```python
from build123d import *

# Parameters (mm, degrees)
SALIENTE_EXTRUIR1_DEPTH = 400
REDONDEO1_R             = 0.5
CROQUIS2_R              = 2
CROQUIS2_R_2            = 1.75
CORTAR_EXTRUIR1_DEPTH   = 16


with BuildPart() as part:
    # Croquis1 → Saliente-Extruir1 (new body)
    with BuildSketch(Plane.XY):
        Polygon((-7.5, 15), (-7.5, 0), (7.5, 0), (7.5, 15), (5.5, 15), (5.5, 2), (-5.5, 2), (-5.5, 15), align=None)
    extrude(amount=SALIENTE_EXTRUIR1_DEPTH)

    # Redondeo1
    redondeo1_edges = [part.edges().sort_by_distance(p)[0] for p in [
        (7.5, 0, 200),
        (-7.5, 0, 200),
    ]]
    fillet(redondeo1_edges, radius=REDONDEO1_R)

    # Croquis2 → Cortar-Extruir1 (cut, through all)
    with BuildSketch(Plane.XZ):
        with Locations((0, 280)):
            Circle(CROQUIS2_R)
        with Locations((0, 330)):
            Circle(CROQUIS2_R)
        with Locations((0, 390)):
            Circle(CROQUIS2_R_2)
        with Locations((0, 380)):
            Circle(CROQUIS2_R_2)
        with Locations((0, 10)):
            Circle(CROQUIS2_R_2)
        with Locations((0, 20)):
            Circle(CROQUIS2_R_2)
        with Locations((0, 230)):
            Circle(CROQUIS2_R)
        with Locations((0, 180)):
            Circle(CROQUIS2_R)
        with Locations((0, 130)):
            Circle(CROQUIS2_R)
        with Locations((0, 80)):
            Circle(CROQUIS2_R)
        with Locations((0, 30)):
            Circle(CROQUIS2_R)
    extrude(amount=-CORTAR_EXTRUIR1_DEPTH, mode=Mode.SUBTRACT)


solid = part.part
```
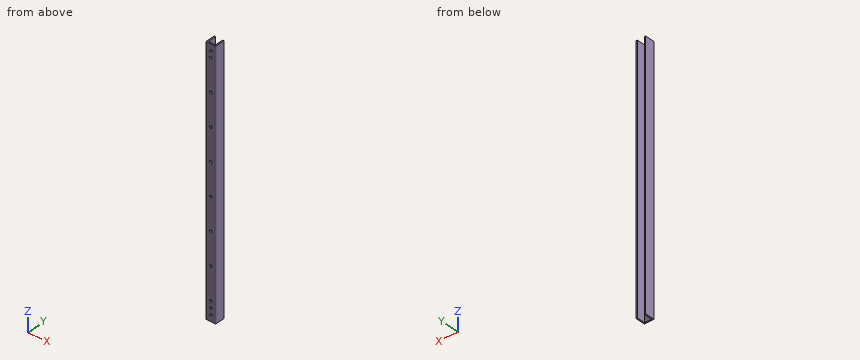
Could you check a few things on this model? Use its own coordinates, in mm. Round coordinates to 2 decimals unless told otherwise and drop trailing zeros. Loops run counter-clockwise (first coordinate to the right, second up) from the corner with the lowest first, then second, coordinate; pieces in that order, holes last. Notation, with made-up numbers: M -23.75,-16.5 L 15.25,-16.5 A17 cw 15.25,-5.5 Z; hole C 30,-5.5 d4. An arc over 180 degrees is marked long. Answer as CSV lines item,"result".
1) If I drill on probe 1 along X at (y, z) = (2.75, 34); probe 2 along X at (y, z) = (0.9, 380); probe 3 along Y at (x, z) = (-2, 207.5), over which ranges is the centre line in solid material (lowest first)?
From the geometry:
probe 1,"-7.5 to -5.5, 5.5 to 7.5"
probe 2,"-7.5 to -1.75, 1.75 to 7.5"
probe 3,"0 to 2"
2) For pin 1 Ø6.5 at (x, z) = (0, 130) entering from +Y, with a flat end and sliding along its axis, tell me the tip position at first contact or that it passes through.
From the geometry:
pin 1,"y = 2"
3) Imagine slicing it at A-A on y = 7. List the corners of the cut face in (x, z) for me.
From the geometry:
outline,"M -7.5,0 L -5.5,0 L -5.5,400 L -7.5,400 Z; M 5.5,0 L 7.5,0 L 7.5,400 L 5.5,400 Z"
4) Imagine slicing it at B-B on z = 290.5. List the corners of the cut face in (x, y) for me, and give its area (3 significant figures).
From the geometry:
outline,"M -7.5,0.5 A0.5 ccw -7,0 L 7,0 A0.5 ccw 7.5,0.5 L 7.5,15 L 5.5,15 L 5.5,2 L -5.5,2 L -5.5,15 L -7.5,15 Z"
area,"81.9 mm^2"
